from build123d import *

# Parameters (mm, degrees)
SKETCH1_W            = 76.2
SKETCH1_H            = 139.7
EXTRUDE1_DEPTH       = 3.175
EXTRUDE2_DEPTH       = 4.175
SKETCH3_W            = 12.7
SKETCH3_H            = 3.175
EXTRUDE3_DEPTH       = 4.175
LPATTERN1_COUNT      = 2
LPATTERN1_PITCH      = 38.1
LPATTERN1_COUNT_DIR2 = 2
LPATTERN1_PITCH_DIR2 = 5.842
SKETCH4_W            = 3.175
SKETCH4_H            = 12.7
EXTRUDE4_DEPTH       = 4.175
LPATTERN2_COUNT      = 3
LPATTERN2_PITCH      = 50.8
LPATTERN2_COUNT_DIR2 = 2
LPATTERN2_PITCH_DIR2 = 66.675


with BuildPart() as part:
    # Sketch1 → Extrude1 (new body)
    with BuildSketch(Plane.XY):
        with Locations((38.1, 69.85)):
            Rectangle(SKETCH1_W, SKETCH1_H)
    extrude(amount=EXTRUDE1_DEPTH)

    # Sketch2 → Extrude2 (cut, through all)
    with BuildSketch(Plane.XY.offset(3.175)):
        with BuildLine():
            Line((40.64, 6.35), (40.64, -24.177687884))
            ThreePointArc((40.64, -24.177687884), (38.1, -26.717687884), (35.56, -24.177687884))
            Line((35.56, -24.177687884), (35.56, 6.35))
            ThreePointArc((35.56, 6.35), (38.1, 8.89), (40.64, 6.35))
        make_face()
    extrude(amount=-EXTRUDE2_DEPTH, mode=Mode.SUBTRACT)

    # Sketch3 → Extrude3 (cut, through all)
    with BuildSketch(Plane.XY.offset(3.175)):
        with Locations((19.05, 23.8125)):
            Rectangle(SKETCH3_W, SKETCH3_H)
    extrude3 = extrude(amount=-EXTRUDE3_DEPTH, mode=Mode.SUBTRACT)

    # LPattern1: Extrude3 2 × 2
    with Locations(*[(i * LPATTERN1_PITCH, -j * LPATTERN1_PITCH_DIR2, 0) for i in range(LPATTERN1_COUNT) for j in range(LPATTERN1_COUNT_DIR2) if (i, j) != (0, 0)]):
        add(extrude3, mode=Mode.SUBTRACT)

    # Sketch4 → Extrude4 (cut, through all)
    with BuildSketch(Plane.XY.offset(3.175)):
        with Locations((71.4375, 6.35)):
            Rectangle(SKETCH4_W, SKETCH4_H)
    extrude4 = extrude(amount=-EXTRUDE4_DEPTH, mode=Mode.SUBTRACT)

    # LPattern2: Extrude4 3 × 2
    with Locations(*[(-j * LPATTERN2_PITCH_DIR2, i * LPATTERN2_PITCH, 0) for i in range(LPATTERN2_COUNT) for j in range(LPATTERN2_COUNT_DIR2) if (i, j) != (0, 0)]):
        add(extrude4, mode=Mode.SUBTRACT)


solid = part.part
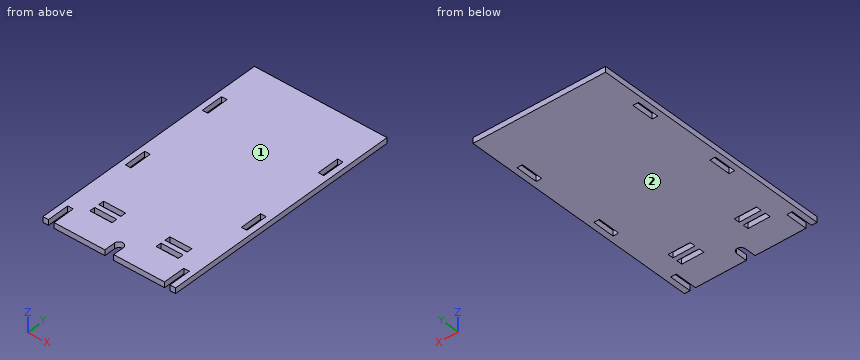
Model file for the job. Use its own axes, mm. Face numbers are marked on the shaded views. Round coordinates to 2 decimals unless told otherwise and drop trailing zeros. Order: outer loops, then holes, each group sorted by start corner. A loop starts at its lowest first (then second) coordinate and runs counter-clockwise, first axis right, second up.
(1) Band-saw the part on C-C (z = 2.45). Give the number of separate pieces and of enclosed holes in the cut face, then the cut area to 3 significant figures.
(2) Band-saw the part on A-A (x = 23). List the corners of the cut face in (y, z) (3 decimals).
(3) Band-saw the part on D-D (x = 38.1). List the corners of the cut face in (y, z) (3 decimals), then the cut area to 3 significant figures.
(4) Pull direction Z, two halves, no side cores. Call the marked faces 1 and 2: released by +Z, released by -Z, zero draft, split by the parting line, or undercut.
(5) Band-saw the part on B-B (y = 54.5). List the corners of the cut face in (x, z) (3 decimals).
(6) Drill centre lines: line 1 (Y direction, x = 23, z = 2.9) (3 decimals); line 2 (X direction, y = 18.5, z = 2.65); line 3 (X direction, y = 105, z = 2) (3 decimals). Where is each one in solid material? Low to high.
Verdict:
1. separate pieces: 1
1. enclosed holes: 8
1. area: 10,200 mm2
2. outline: (0, 0) - (16.383, 0) - (16.383, 3.175) - (0, 3.175) - close; (19.558, 0) - (22.225, 0) - (22.225, 3.175) - (19.558, 3.175) - close; (25.4, 0) - (139.7, 0) - (139.7, 3.175) - (25.4, 3.175) - close
3. outline: (8.89, 0) - (139.7, 0) - (139.7, 3.175) - (8.89, 3.175) - close
3. area: 415 mm2
4. face 1: released by +Z
4. face 2: released by -Z
5. outline: (0, 0) - (3.175, 0) - (3.175, 3.175) - (0, 3.175) - close; (6.35, 0) - (69.85, 0) - (69.85, 3.175) - (6.35, 3.175) - close; (73.025, 0) - (76.2, 0) - (76.2, 3.175) - (73.025, 3.175) - close
6. line 1: y = 0 to 16.383, 19.558 to 22.225, 25.4 to 139.7
6. line 2: x = 0 to 12.7, 25.4 to 50.8, 63.5 to 76.2
6. line 3: x = 0 to 3.175, 6.35 to 69.85, 73.025 to 76.2
